Check sheet for the modelled part. Datum: model origin and axes. Units: mm. A direction names the side the tool comes from. Give positions to 0.01 mm unless a question says otherwise; leave off trailing zeros. Order: outer loops, then holes, each group sorted by start corner. A loop starts at its lowest first (then second) coordinate and runs counter-clockwise, first axis right, second up.
Item 1: Gauge pin test, flat ends, axial feed: P1, Ø13, axis at y = 73.5, z = 1, coming from the +X side; P2, Ø5, axis at x = 34, y = 76.5, coming from the -Z side; P3, Ø11, axis at x = 33, y = 81, coming from the +Z side; P4, Ø12, axis at x = 18, z = 11, coming from the -Y side. Record the tip position at first contact, or that the pin passes through.
Item 2: Release check for a two-part mould opening along Z. For faces 5 (the flat face through (13, 49.3, -5.7)), 6 (the flat face through (30, 74, -8)), 7 (the flat face through (25, 10, -19)) record: released by +Z, released by -Z, zero draft, split by the parting line, or undercut.
Item 3: Sectioned sample at B-B on x = 35.5. Record the boundary of the cut face in (y, z).
Item 4: Material ranges on line 1 along X through (y, z) = (16.5, 0); line 2 along Z through (x, y) = (34, 76); line 3 along X through (y, z) = (65.5, -2), recorded low to high.
Item 5: Sectioned sample at A-A on z = 0. Record the boundary of the cut face in (x, y), and give its area (3 significant figures).
Item 6: Sectioned sample at C-C on y = 85. Record the boundary of the cut face in (x, z).
Item 7: Access from +Z, -Z, +X, -X, +Y, -Y to the whole of each face (thin tool, end or side, straight path). Record for faces 1 (the flat face through (25, 75, 19)), 2 (the flat face through (25, 75, -19)), 3 (the flat face through (30, 74, 8)), 4 (the flat face through (23, 74, 0)).
Item 8: Sectioned sample at D-D on z = -13.5. Record the boundary of the cut face in (x, y), and give its area (3 significant figures).
from build123d import *

# Parameters (mm, degrees)
F0_W      = 24
F0_H      = 38
F1_DEPTH  = 100
F3_R      = 24
F4_DEPTH  = 24
F5_R      = 15
F6_DEPTH  = 25
F7_DEPTH  = 25
F9_DEPTH  = 14
F10_DEPTH = 25
F11_R     = 9
F12_DEPTH = 25


with BuildPart() as f1:
    # F0 (on Front) → F1 (new body)
    with BuildSketch(Plane.XZ):
        Rectangle(F0_W, F0_H)
    extrude(amount=-F1_DEPTH)

    # F3 (on face) → F4 (join)
    with BuildSketch(Plane.YZ.offset(12)):
        with Locations((35.1973697543, 0)):
            Circle(F3_R)
    extrude(amount=-F4_DEPTH)

    # F5 (on face) → F6 (cut)
    with BuildSketch(Plane.YZ.offset(12)):
        with Locations((35.1973697543, 0)):
            Circle(F5_R)
    extrude(amount=-F6_DEPTH, mode=Mode.SUBTRACT)

    # F7 (add): a face of the model
    f7_faces = [f1.faces().sort_by_distance(p)[0] for p in [
        (12, 52.2784311764, 0),
    ]]
    extrude(f7_faces, amount=F7_DEPTH)

    # F8 (on face) → F9 (cut)
    with BuildSketch(Plane.YZ.offset(37)):
        with BuildLine():
            Line((47.8859472948, -8), (100, -8))
            Line((100, -8), (100, 8))
            Line((100, 8), (47.8859472948, 8))
            ThreePointArc((47.8859472948, 8), (49.6079329478, 4.1636124275), (50.1973697543, 0))
            ThreePointArc((50.1973697543, 0), (49.6079329478, -4.1636124275), (47.8859472948, -8))
        make_face()
    extrude(amount=-F9_DEPTH, mode=Mode.SUBTRACT)

    # F10 (cut): a face of the model
    f10_faces = [f1.faces().sort_by_distance(p)[0] for p in [
        (-12, 52.2784311764, 0),
    ]]
    extrude(f10_faces, amount=-F10_DEPTH, mode=Mode.SUBTRACT)

    # F11 (on face) → F12 (cut)
    with BuildSketch(Plane.XZ):
        with Locations((25.1644738019, 0)):
            Circle(F11_R)
    extrude(amount=-F12_DEPTH, mode=Mode.SUBTRACT)


solid = f1.part
Report:
1. P1: stops at x = 23
1. P2: stops at z = -19
1. P3: stops at z = 19
1. P4: stops at y = 0
2. face 5: zero draft
2. face 6: undercut
2. face 7: released by -Z
3. outline: (0, -19) - (20.53, -19) arc R24 ccw to (49.86, -19) - (100, -19) - (100, -8) - (47.89, -8) arc R15 cw (long way) to (47.89, 8) - (100, 8) - (100, 19) - (49.86, 19) arc R24 ccw to (20.53, 19) - (0, 19) - close
4. line 1: x = 13 to 16.16, 34.16 to 37
4. line 2: z = -19 to -8, 8 to 19
4. line 3: x = 13 to 23
5. outline: (13, 0) - (16.16, 0) - (16.16, 20.2) - (13, 20.2) - close; (13, 50.2) - (23, 50.2) - (23, 100) - (13, 100) - close; (34.16, 0) - (37, 0) - (37, 20.2) - (34.16, 20.2) - close
5. area: 619 mm2
6. outline: (13, -19) - (37, -19) - (37, -8) - (23, -8) - (23, 8) - (37, 8) - (37, 19) - (13, 19) - close
7. face 1: +Z, +X, -X, +Y
7. face 2: -Z, +X, -X, +Y
7. face 3: +X, +Y
7. face 4: +X, +Y, -Y
8. outline: (13, 0) - (37, 0) - (37, 28.66) - (13, 28.66) - close; (13, 41.74) - (37, 41.74) - (37, 100) - (13, 100) - close
8. area: 2,090 mm2
